Could you check a few things on this model? Use its own coordinates, in mm. Face numbers are marked on the shaded views. A direction names the side the tool comes from. Coordinates: 2 decimals unless noted, no trailing zeros. Loops run counter-clockwise (first coordinate to the right, second up) from the corner with the lowest first, then second, coordinate; pieces in that order, holes last. Notation, with made-up numbers: M -31,62 L 16,62 A17 cw 16,92 Z; hole C 43.25,26 d10. An arc over 180 degrees is marked long. Return JSON: item names as keys, results as strings. Group by question number.
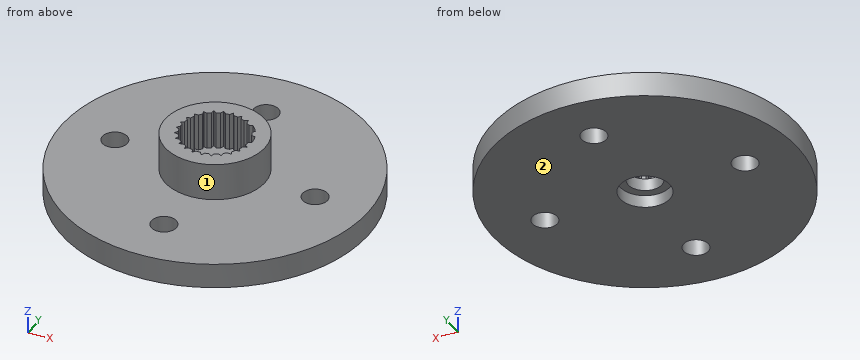
from build123d import *

# Parameters (mm, degrees)
SKETCH1_R           = 12.25
BOSS_EXTRUDE1_DEPTH = 2
SKETCH2_R           = 1
CUT_EXTRUDE1_DEPTH  = 2
SKETCH3_R           = 1.35
CUT_EXTRUDE2_DEPTH  = 4
SKETCH4_R           = 4
SKETCH4_R_2         = 2.88
BOSS_EXTRUDE2_DEPTH = 3
SKETCH6_R           = 2
CUT_EXTRUDE3_DEPTH  = 1
BOSS_EXTRUDE4_START = -3
BOSS_EXTRUDE4_DEPTH = 3


with BuildPart() as part:
    # Sketch1 → Boss-Extrude1 (new body)
    with BuildSketch(Plane.XY):
        Circle(SKETCH1_R)
    extrude(amount=BOSS_EXTRUDE1_DEPTH)

    # Sketch2 → Cut-Extrude1 (cut)
    with BuildSketch(Plane.XY.offset(2)):
        with Locations((-8, 0)):
            Circle(SKETCH2_R)
        with Locations((0, 8)):
            Circle(SKETCH2_R)
        with Locations((8, 0)):
            Circle(SKETCH2_R)
        with Locations((0, -8)):
            Circle(SKETCH2_R)
    extrude(amount=-CUT_EXTRUDE1_DEPTH, mode=Mode.SUBTRACT)

    # Sketch3 → Cut-Extrude2 (cut)
    with BuildSketch(Plane.XY.offset(2)):
        Circle(SKETCH3_R)
    extrude(amount=-CUT_EXTRUDE2_DEPTH, mode=Mode.SUBTRACT)

    # Sketch4 → Boss-Extrude2 (add)
    with BuildSketch(Plane.XY.offset(2)):
        Circle(SKETCH4_R)
        Circle(SKETCH4_R_2, mode=Mode.SUBTRACT)
    extrude(amount=BOSS_EXTRUDE2_DEPTH)

    # Sketch6 → Cut-Extrude3 (cut)
    with BuildSketch(Plane(origin=(0, 0, 0), x_dir=(-1, 0, 0), z_dir=(0, 0, -1))):
        Circle(SKETCH6_R)
    extrude(amount=-CUT_EXTRUDE3_DEPTH, mode=Mode.SUBTRACT)

    # Sketch5 → Boss-Extrude4 (add)
    with BuildSketch(Plane.XY.offset(5).offset(BOSS_EXTRUDE4_START)):
        with BuildLine():
            Line((-0.161756527, -2.620613729), (-0.351910166, -2.85841901))
            ThreePointArc((-0.351910166, -2.85841901), (0.000368858, -2.879999976), (0.352642342, -2.858328774))
            Line((0.352642342, -2.858328774), (0.162522941, -2.62056631))
            ThreePointArc((0.162522941, -2.62056631), (0.00038394, -2.625601139), (-0.161756527, -2.620613729))
        make_face()
        with BuildLine():
            ThreePointArc((-1.051714162, -2.681100021), (-0.715869599, -2.789611212), (-0.369274025, -2.856227703))
            Line((-0.369274025, -2.856227703), (-0.494291356, -2.578654212))
            ThreePointArc((-0.494291356, -2.578654212), (-0.652588574, -2.543208533), (-0.808394781, -2.498055117))
            Line((-0.808394781, -2.498055117), (-1.051714162, -2.681100021))
        make_face()
        with BuildLine():
            Line((0.495045485, -2.578509542), (0.37000564, -2.85613302))
            ThreePointArc((0.37000564, -2.85613302), (0.716584139, -2.78942775), (1.052400895, -2.680830535))
            Line((1.052400895, -2.680830535), (0.809125323, -2.497818589))
            ThreePointArc((0.809125323, -2.497818589), (0.653332329, -2.54301757), (0.495045485, -2.578509542))
        make_face()
        with BuildLine():
            ThreePointArc((-1.685435089, -2.335317657), (-1.387127337, -2.523940917), (-1.067987548, -2.674659342))
            Line((-1.067987548, -2.674659342), (-1.12004751, -2.374715787))
            ThreePointArc((-1.12004751, -2.374715787), (-1.264556547, -2.301016782), (-1.404238617, -2.218534516))
            Line((-1.404238617, -2.218534516), (-1.685435089, -2.335317657))
        make_face()
        with BuildLine():
            Line((1.120741967, -2.374388118), (1.068672631, -2.674385688))
            ThreePointArc((1.068672631, -2.674385688), (1.387773803, -2.523585519), (1.686033229, -2.334885854))
            Line((1.686033229, -2.334885854), (1.404887387, -2.218123739))
            ThreePointArc((1.404887387, -2.218123739), (1.265229445, -2.300646853), (1.120741967, -2.374388118))
        make_face()
        with BuildLine():
            ThreePointArc((-2.213253931, -1.842798696), (-1.971226763, -2.09968213), (-1.699595485, -2.325032298))
            Line((-1.699595485, -2.325032298), (-1.675426958, -2.021565235))
            ThreePointArc((-1.675426958, -2.021565235), (-1.797067781, -1.914243684), (-1.911848977, -1.799615231))
            Line((-1.911848977, -1.799615231), (-2.213253931, -1.842798696))
        make_face()
        with BuildLine():
            Line((1.676018111, -2.021075155), (1.70019099, -2.324596868))
            ThreePointArc((1.70019099, -2.324596868), (1.971764535, -2.099177129), (2.213725894, -1.842231708))
            Line((2.213725894, -1.842231708), (1.912375208, -1.799056017))
            ThreePointArc((1.912375208, -1.799056017), (1.797627541, -1.913718034), (1.676018111, -2.021075155))
        make_face()
        with BuildLine():
            ThreePointArc((-2.602005889, -1.234489916), (-2.431466761, -1.543492594), (-2.224411588, -1.829314923))
            Line((-2.224411588, -1.829314923), (-2.12553317, -1.541392304))
            ThreePointArc((-2.12553317, -1.541392304), (-2.216662638, -1.407191614), (-2.299330835, -1.267619503))
            Line((-2.299330835, -1.267619503), (-2.602005889, -1.234489916))
        make_face()
        with BuildLine():
            Line((2.125983872, -1.540770608), (2.224880096, -1.828745077))
            ThreePointArc((2.224880096, -1.828745077), (2.43186205, -1.54286972), (2.60232202, -1.233823368))
            Line((2.60232202, -1.233823368), (2.299701462, -1.26694699))
            ThreePointArc((2.299701462, -1.26694699), (2.217074088, -1.406543272), (2.125983872, -1.540770608))
        make_face()
        with BuildLine():
            ThreePointArc((-2.827264247, -0.548613595), (-2.738928761, -0.890319741), (-2.609459729, -1.218654964))
            Line((-2.609459729, -1.218654964), (-2.442084315, -0.964368026))
            ThreePointArc((-2.442084315, -0.964368026), (-2.496976429, -0.811720521), (-2.542337279, -0.655974579))
            Line((-2.542337279, -0.655974579), (-2.827264247, -0.548613595))
        make_face()
        with BuildLine():
            Line((2.442366248, -0.963653777), (2.609771804, -1.217986508))
            ThreePointArc((2.609771804, -1.217986508), (2.739156728, -0.889618132), (2.827404683, -0.547889369))
            Line((2.827404683, -0.547889369), (2.542529016, -0.655231023))
            ThreePointArc((2.542529016, -0.655231023), (2.497213717, -0.810990224), (2.442366248, -0.963653777))
        make_face()
        with BuildLine():
            ThreePointArc((-2.874875195, 0.171734137), (-2.874293794, -0.181204825), (-2.830545919, -0.531422432))
            Line((-2.830545919, -0.531422432), (-2.605190321, -0.326748959))
            ThreePointArc((-2.605190321, -0.326748959), (-2.620396008, -0.165246042), (-2.625599323, -0.00311236))
            Line((-2.625599323, -0.00311236), (-2.874875195, 0.171734137))
        make_face()
        with BuildLine():
            Line((2.60528577, -0.325987035), (2.830681951, -0.530697366))
            ThreePointArc((2.830681951, -0.530697366), (2.874340115, -0.180468565), (2.874831111, 0.172470535))
            Line((2.874831111, 0.172470535), (2.625600121, -0.002344481))
            ThreePointArc((2.625600121, -0.002344481), (2.620444223, -0.164479678), (2.60528577, -0.325987035))
        make_face()
        with BuildLine():
            ThreePointArc((-2.741847161, 0.881291181), (-2.829056376, 0.539295857), (-2.873778498, 0.189201326))
            Line((-2.873778498, 0.189201326), (-2.604602638, 0.331400948))
            ThreePointArc((-2.604602638, 0.331400948), (-2.579166468, 0.491611454), (-2.543885305, 0.64994542))
            Line((-2.543885305, 0.64994542), (-2.741847161, 0.881291181))
        make_face()
        with BuildLine():
            ThreePointArc((-2.436538786, 1.535473459), (-2.606058942, 1.225910597), (-2.736441006, 0.897936869))
            Line((-2.736441006, 0.897936869), (-2.440358193, 0.968727714))
            ThreePointArc((-2.440358193, 0.968727714), (-2.375878414, 1.117579194), (-2.302329617, 1.262164738))
            Line((-2.302329617, 1.262164738), (-2.436538786, 1.535473459))
        make_face()
        with BuildLine():
            ThreePointArc((-1.978133718, 2.093176293), (-2.21931324, 1.835496865), (-2.427162861, 1.550251736))
            Line((-2.427162861, 1.550251736), (-2.122777067, 1.545185755))
            ThreePointArc((-2.122777067, 1.545185755), (-2.023305181, 1.673325323), (-1.916110092, 1.795077605))
            Line((-1.916110092, 1.795077605), (-1.978133718, 2.093176293))
        make_face()
        with BuildLine():
            Line((2.440995413, 0.967120926), (2.73696806, 0.89632909))
            ThreePointArc((2.73696806, 0.89632909), (2.605878342, 1.226294446), (2.435183429, 1.537622082))
            Line((2.435183429, 1.537622082), (2.282024688, 1.298516389))
            ThreePointArc((2.282024688, 1.298516389), (2.367316087, 1.135603819), (2.440995413, 0.967120926))
        make_face()
        with BuildLine():
            ThreePointArc((-1.395435234, 2.519357162), (-1.693119925, 2.329752115), (-1.965377147, 2.105158585))
            Line((-1.965377147, 2.105158585), (-1.671814051, 2.024554092))
            ThreePointArc((-1.671814051, 2.024554092), (-1.543600242, 2.123930268), (-1.409494323, 2.215199143))
            Line((-1.409494323, 2.215199143), (-1.395435234, 2.519357162))
        make_face()
        with BuildLine():
            ThreePointArc((-0.725056422, 2.787237554), (-1.060541659, 2.677620472), (-1.380099559, 2.527790578))
            Line((-1.380099559, 2.527790578), (-1.115804809, 2.37671225))
            ThreePointArc((-1.115804809, 2.37671225), (-0.966905223, 2.441080863), (-0.814314842, 2.496131573))
            Line((-0.814314842, 2.496131573), (-0.725056422, 2.787237554))
        make_face()
        with BuildLine():
            ThreePointArc((-0.009119648, 2.879985561), (-0.361325659, 2.857244086), (-0.70810524, 2.791592192))
            Line((-0.70810524, 2.791592192), (-0.489685448, 2.579532836))
            ThreePointArc((-0.489685448, 2.579532836), (-0.329455993, 2.60484937), (-0.167968964, 2.620222876))
            Line((-0.167968964, 2.620222876), (-0.009119648, 2.879985561))
        make_face()
        with BuildLine():
            Line((1.671221881, 2.025042942), (1.964837844, 2.10566195))
            ThreePointArc((1.964837844, 2.10566195), (1.6925231, 2.330185734), (1.394789851, 2.519714522))
            Line((1.394789851, 2.519714522), (1.408846409, 2.215611267))
            ThreePointArc((1.408846409, 2.215611267), (1.542979014, 2.124381616), (1.671221881, 2.025042942))
        make_face()
        with BuildLine():
            ThreePointArc((0.707390147, 2.791773483), (0.36059376, 2.857336547), (0.008381935, 2.879987803))
            Line((0.008381935, 2.879987803), (0.167202651, 2.620271888))
            ThreePointArc((0.167202651, 2.620271888), (0.328694169, 2.604945611), (0.488931021, 2.579675939))
            Line((0.488931021, 2.579675939), (0.707390147, 2.791773483))
        make_face()
        with BuildLine():
            Line((1.115109672, 2.377038475), (1.379452017, 2.52814401))
            ThreePointArc((1.379452017, 2.52814401), (1.059855747, 2.677892043), (0.724342443, 2.787423187))
            Line((0.724342443, 2.787423187), (0.813584792, 2.49636962))
            ThreePointArc((0.813584792, 2.49636962), (0.966191267, 2.441363538), (1.115109672, 2.377038475))
        make_face()
    extrude(amount=BOSS_EXTRUDE4_DEPTH)


solid = part.part
(1) Imagine slicing it at B-B, the plane z = 1.6. Write out the boundary of the cut face in (x, y).
(2) Imagine slicing it at D-D, the plane x = -4.5. Write out the boundary of the cut face in (y, z).
(3) Imagine slicing it at A-A, the plane x = -8. Write out the boundary of the cut face in (y, z).
(4) Will these pins go through, and if not, where does the flat tip stop? P1, Ø3, axis at x = 0, y = 0, coming from the -Z side; P2, Ø3, axis at x = 0, y = 8, coming from the +Z side; P3, Ø3, axis at x = 0, y = -8, coming from the -Z side; P4, Ø1.5, axis at y = 7, z = 2, coming from the +X side.
(5) If I drill on L1, parallel to Y at x = 0, z = 1.7; L2, parallel to Y at x = 0, z = 0.6; L3, parallel to Z at x = -9.25, y = -3.75, over which ranges is the centre line in solid material (lowest first)? Write a range as [from, to].
(6) For the marked faces 1 and 2, which set-ups out of +Z, -Z, +X, -X, +Y, -Y let a thin tool reach every point of the face, with its end or its side?
Checks:
{
 "1": {"outline": "C 0,0 d24.5; hole C -8,0 d2; hole C 0,0 d2.7; hole C 0,-8 d2; hole C 0,8 d2; hole C 8,0 d2"},
 "2": {"outline": "M -11.39,0 L 11.39,0 L 11.39,2 L -11.39,2 Z"},
 "3": {"outline": "M -9.28,0 L -1,0 L -1,2 L -9.28,2 Z; M 1,0 L 9.28,0 L 9.28,2 L 1,2 Z"},
 "4": {"P1": "z = 1", "P2": "z = 2", "P3": "z = 0", "P4": "x = 10.54"},
 "5": {"L1": "[-12.25, -9], [-7, -1.35], [1.35, 7], [9, 12.25]", "L2": "[-12.25, -9], [-7, -2], [2, 7], [9, 12.25]", "L3": "[0, 2]"},
 "6": {"face 1": "+Z", "face 2": "-Z, +X, -X, +Y, -Y"}
}
